from build123d import *

# Parameters (mm, degrees)
SKETCH2_R           = 75
BOSS_EXTRUDE2_DEPTH = 10
SKETCH1_R           = 8
CUT_EXTRUDE2_DEPTH  = 10


with BuildPart() as part:
    # Sketch2 → Boss-Extrude2 (new body)
    with BuildSketch(Plane(origin=(0, 0, 0), x_dir=(1, 0, 0), z_dir=(0, 1, 0))):
        with Locations(Location((0, 0, 0), (0, 0, 270))):
            Circle(SKETCH2_R)
    extrude(amount=BOSS_EXTRUDE2_DEPTH)

    # Sketch1 → Cut-Extrude2 (cut)
    with BuildSketch(Plane(origin=(0, 0, 0), x_dir=(1, 0, 0), z_dir=(0, 1, 0))):
        with Locations(Location((-1.432800613, 0, 0), (0, 0, 270))):
            Circle(SKETCH1_R)
        with BuildLine():
            Line((-35.952412724, 6.579299902), (-29.089373403, 6.579299902))
            add(Edge.make_bspline(
                [(-29.089373403, 6.579299902), (-27.025622413, -9.672081056), (-24.297966674, -7.419579117), (-18.166448585, -14.521920914)],
                knots=[0, 0, 0, 0, 1, 1, 1, 1], degree=3))
            add(Edge.make_bspline(
                [(-18.166448585, -14.521920914), (-13.477906245, -22.059485723), (-13.054308641, -27.941832091), (-13.424345656, -40.15305356)],
                knots=[0, 0, 0, 0, 1, 1, 1, 1], degree=3))
            Line((-13.424345656, -40.15305356), (-8.687329727, -40.15305356))
            Line((-8.687329727, -40.15305356), (-8.687329727, -15.15305356))
            Line((-8.687329727, -15.15305356), (-20.216966385, 4.843209587))
            ThreePointArc((-20.216966385, 4.843209587), (-22.512806675, 10.333533655), (-17.90159089, 6.571721593))
            Line((-17.90159089, 6.571721593), (-5.592864867, -10.764187934))
            Line((-5.592864867, -10.764187934), (2.72726364, -10.764187934))
            Line((2.72726364, -10.764187934), (15.035989663, 6.571721593))
            ThreePointArc((15.035989663, 6.571721593), (19.647205448, 10.333533655), (17.351365158, 4.843209587))
            Line((17.351365158, 4.843209587), (5.8217285, -15.15305356))
            Line((5.8217285, -15.15305356), (5.8217285, -40.15305356))
            Line((5.8217285, -40.15305356), (10.558744429, -40.15305356))
            add(Edge.make_bspline(
                [(15.300847358, -14.521920914), (10.612305018, -22.059485723), (10.188707415, -27.941832091), (10.558744429, -40.15305356)],
                knots=[0, 0, 0, 0, 1, 1, 1, 1], degree=3))
            add(Edge.make_bspline(
                [(26.223772176, 6.579299902), (24.160021186, -9.672081056), (21.432365448, -7.419579117), (15.300847358, -14.521920914)],
                knots=[0, 0, 0, 0, 1, 1, 1, 1], degree=3))
            Line((26.223772176, 6.579299902), (33.086811497, 6.579299902))
            add(Edge.make_bspline(
                [(33.086811497, 6.579299902), (34.136872369, -13.750794086), (20.402844412, -15.135742794), (17.812300069, -27.718386748)],
                knots=[0, 0, 0, 0, 1, 1, 1, 1], degree=3))
            Line((17.812300069, -27.718386748), (17.812300069, -46.666450461))
            Line((17.812300069, -46.666450461), (-0.691668401, -46.666450461))
            Line((-0.691668401, -46.666450461), (-0.691668401, -30.679021703))
            Line((-0.691668401, -30.679021703), (-1.432800613, -30.679021703))
            Line((-1.432800613, -30.679021703), (-2.173932826, -30.679021703))
            Line((-2.173932826, -30.679021703), (-2.173932826, -46.666450461))
            Line((-2.173932826, -46.666450461), (-20.677901296, -46.666450461))
            Line((-20.677901296, -46.666450461), (-20.677901296, -27.718386748))
            add(Edge.make_bspline(
                [(-35.952412724, 6.579299902), (-37.002473596, -13.750794086), (-23.268445639, -15.135742794), (-20.677901296, -27.718386748)],
                knots=[0, 0, 0, 0, 1, 1, 1, 1], degree=3))
        make_face()
        with BuildLine():
            Line((-31.134175081, 56.453740846), (-24.814846439, 46.586253524))
            ThreePointArc((-24.814846439, 46.586253524), (-21.361233135, 45.829579865), (-20.604559476, 49.283193168))
            Line((-20.604559476, 49.283193168), (-26.984364124, 59.240747711))
            ThreePointArc((-26.984364124, 59.240747711), (-30.483201963, 59.96745797), (-31.134175081, 56.453740846))
        make_face()
        with BuildLine():
            Line((-13.424345656, -48.522506104), (11.473739755, -48.522506104))
            ThreePointArc((11.473739755, -48.522506104), (14.973739755, -52.022506104), (11.473739755, -55.522506104))
            Line((11.473739755, -55.522506104), (-13.424345656, -55.522506104))
            ThreePointArc((-13.424345656, -55.522506104), (-16.924345656, -52.022506104), (-13.424345656, -48.522506104))
        make_face()
        with BuildLine():
            Line((-11.201579128, -56.280200871), (9.314578626, -56.280200871))
            ThreePointArc((9.314578626, -56.280200871), (12.614578626, -59.580200871), (9.314578626, -62.880200871))
            Line((9.314578626, -62.880200871), (-11.201579128, -62.880200871))
            ThreePointArc((-11.201579128, -62.880200871), (-14.501579128, -59.580200871), (-11.201579128, -56.280200871))
        make_face()
        with BuildLine():
            Line((-5.872415439, -63.856077067), (3.199630927, -63.856077067))
            ThreePointArc((3.199630927, -63.856077067), (6.199630927, -66.856077067), (3.199630927, -69.856077067))
            Line((3.199630927, -69.856077067), (-5.872415439, -69.856077067))
            ThreePointArc((-5.872415439, -69.856077067), (-8.872415439, -66.856077067), (-5.872415439, -63.856077067))
        make_face()
        with BuildLine():
            Line((1.332228572, 52.068816937), (1.332228572, 64.224401135))
            ThreePointArc((1.332228572, 64.224401135), (-1.167771428, 66.724401135), (-3.667771428, 64.224401135))
            Line((-3.667771428, 64.224401135), (-3.667771428, 52.068816937))
            ThreePointArc((-3.667771428, 52.068816937), (-1.167771428, 49.568816937), (1.332228572, 52.068816937))
        make_face()
        with BuildLine():
            Line((17.812300069, 47.984100232), (24.687796247, 58.598066559))
            ThreePointArc((24.687796247, 58.598066559), (28.150603832, 59.333538892), (28.877039625, 55.868824335))
            Line((28.877039625, 55.868824335), (22.233533262, 45.729327008))
            ThreePointArc((22.233533262, 45.729327008), (18.749192485, 44.359153526), (17.812300069, 47.984100232))
        make_face()
        with BuildLine():
            Line((38.137038152, 12.721700218), (52.193121227, 12.721700218))
            ThreePointArc((52.193121227, 12.721700218), (54.693121227, 10.221700218), (52.193121227, 7.721700218))
            Line((52.193121227, 7.721700218), (38.137038152, 7.721700218))
            ThreePointArc((38.137038152, 7.721700218), (35.637038152, 10.221700218), (38.137038152, 12.721700218))
        make_face()
        with BuildLine():
            Line((-47.564108381, 39.405649722), (-37.144284237, 33.563931274))
            ThreePointArc((-37.144284237, 33.563931274), (-35.434524966, 30.128871371), (-39.118884044, 29.057231746))
            Line((-39.118884044, 29.057231746), (-50.146349023, 35.309342232))
            ThreePointArc((-50.146349023, 35.309342232), (-51.497079679, 39.022872656), (-47.564108381, 39.405649722))
        make_face()
        with BuildLine():
            Line((-55.264750738, 12.721700218), (-40.570294155, 12.721700218))
            ThreePointArc((-40.570294155, 12.721700218), (-38.070294155, 10.221700218), (-40.570294155, 7.721700218))
            Line((-40.570294155, 7.721700218), (-55.264750738, 7.721700218))
            ThreePointArc((-55.264750738, 7.721700218), (-57.764750738, 10.221700218), (-55.264750738, 12.721700218))
        make_face()
        with BuildLine():
            Line((35.054833416, 33.324298088), (47.015148154, 39.881834455))
            ThreePointArc((47.015148154, 39.881834455), (50.409175042, 38.891591313), (49.4189319, 35.497564425))
            Line((49.4189319, 35.497564425), (37.458617163, 28.940028057))
            ThreePointArc((37.458617163, 28.940028057), (34.064590274, 29.930271199), (35.054833416, 33.324298088))
        make_face()
        with BuildLine():
            ThreePointArc((-33.046716349, 17.625870716), (-33.455059745, 11.692930554), (-31.500963756, 17.309694049))
            ThreePointArc((-31.500963756, 17.309694049), (-26.882220389, 19.905184059), (-27.162966351, 25.195792756))
            ThreePointArc((-27.162966351, 25.195792756), (-22.104048649, 27.055183334), (-21.13695027, 32.357513233))
            ThreePointArc((-21.13695027, 32.357513233), (-14.620111434, 32.395294639), (-11.406386962, 38.06473825))
            ThreePointArc((-11.406386962, 38.06473825), (-4.396601986, 34.681279815), (1.471524132, 39.794984172))
            ThreePointArc((1.471524132, 39.794984172), (6.193027263, 34.08541272), (13.594903675, 34.407939573))
            ThreePointArc((13.594903675, 34.407939573), (16.549089374, 26.949655565), (24.427689797, 25.439401003))
            ThreePointArc((24.427689797, 25.439401003), (33.733708737, 12.53660842), (27.3780871, 27.120507712))
            ThreePointArc((27.3780871, 27.120507712), (28.671886083, 38.175165666), (17.822025263, 40.657079943))
            ThreePointArc((17.822025263, 40.657079943), (11.030714439, 49.871470086), (1.471524132, 43.574743231))
            ThreePointArc((1.471524132, 43.574743231), (-6.400960855, 48.670912402), (-12.400625348, 41.463209157))
            ThreePointArc((-12.400625348, 41.463209157), (-20.931972428, 43.767512306), (-23.888413897, 35.43965845))
            ThreePointArc((-23.888413897, 35.43965845), (-30.449277719, 34.011905286), (-30.611197445, 27.299439629))
            ThreePointArc((-30.611197445, 27.299439629), (-36.148201567, 23.550113394), (-33.046716349, 17.625870716))
        make_face()
    extrude(amount=CUT_EXTRUDE2_DEPTH, mode=Mode.SUBTRACT)


solid = part.part
Work out the finished part from the listing and answer in its coordinate system (mm). Coordinates: 2 decimals unless noted, no trailing zeros. Order: outer loops, then holes, each group sorted by start corner. A loop starts at its lowest first (then second) coordinate and runs counter-clockwise, first axis right, second up. Notation, with made-up numbers: (5, 68.25) - (27, 68.25) arc R29 ccw to (27, 104.25) - close; hole circle Ø5 at (45.5, 77). An arc over 180 degrees is marked (long way). Put each result on its own line as item: value. Start each with the question number.
1) Flat-ended cylindrical pins translate along their axes: pin 1 (1 mm diameter, centred on y = 2.5, z = 33.5, fed in from -X); pin 2 (4 mm diameter, centred on y = 3, z = 58, fed in from -X); pin 3 (3 mm diameter, centred on y = 7, z = -57.5, fed in from +X). Find the tip coordinate at first contact, or state that the pin passes through.
2) Find the intervals of material crossed by line 1 (Z direction, x = -49, y = 5.25); line 2 (X direction, y = 3.75, z = 17); line 3 (X direction, y = 8.5, z = 19.5), in increasing order. Write a range as from..to.
3) Find section B-B (z = 0). State how many separate pieces and enclosed holes the cut face has, plus the area to 3 significant figures.
4) Find section A-A (x = -45.5). Give the vertices of the cut face in (y, z).
Results list:
1. pin 1: stops at x = -67.35
1. pin 2: stops at x = -49.89
1. pin 3: stops at x = 49.89
2. line 1: z = -56.78..-40.16, -34.66..-12.72, -7.72..56.78
2. line 2: x = -73.05..-26.66, -16.75..-8.69, 5.82..13.88, 23.8..73.05
2. line 3: x = -72.42..-24.61, -15.59..-8.69, 5.82..12.72, 21.75..72.42
3. separate pieces: 6
3. enclosed holes: 0
3. area: 1,100 mm^2
4. outline: (0, -59.62) - (10, -59.62) - (10, -38.25) - (0, -38.25) - close; (0, -32.68) - (10, -32.68) - (10, -12.72) - (0, -12.72) - close; (0, -7.72) - (10, -7.72) - (10, 59.62) - (0, 59.62) - close
